Model file for the job. Use its own axes, mm. Face numbers are marked on the shaded views. A direction names the side the tool comes from. Coordinates: 2 decimals unless noted, no trailing zeros. Write each loop counter-clockwise with the first axis right and the second up, starting at its lowest first coordinate (ties: lowest second). Pieces come first, ordered by that corner, then holes.
Q1. Pull direction X, two halves, no side cores. Call the marked faces 5, 6 and 7: released by +X, released by -X, zero draft, split by the parting line, or undercut.
Q2. Band-saw the part on D-D, the plane y = -19.5. Write the cut outline in (x, z).
Q3. Band-saw the part on C-C, the plane x = -13.5. Write the cut outline in (y, z), plus the area to 3 significant figures.
Q4. Band-saw the part on B-B, the plane z = 7.5. Write the cut outline in (x, y).
Q5. Pin check, flat tips, straight feed: P1, Ø14.5, axis at x = -13, y = 9.5, coming from the +Z side; P2, Ø1.5, axis at y = -7, z = 7.5, coming from the +X side; P3, Ø1, axis at x = -4.5, z = 3, coming from the +Y side. Stop position of each tip, or through.
Q6. Band-saw the part on A-A, the plane y = -2.5. Write the cut outline in (x, z), plus the area to 3 significant figures.
Q7. Which spindle directions (+Z, -Z, +X, -X, +Y, -Y) get a long thin tool onto all of the face, cutting with end or side? Do the marked faces 1, 2, 3 and 4. Say none if no direction does.
Q8. Drill centre lines: probe 1 along X at (y, z) = (-3, 1.75); probe 2 along X at (y, z) = (-23, 4.5); probe 3 along Y at (x, z) = (-29.5, 8.5). Where is each one in solid material? Low to high.
from build123d import *

# Parameters (mm, degrees)
F0_W      = 90
F0_H      = 59.1
F0_R      = 1.55
F1_DEPTH  = 1.65
F2_W      = 63
F2_H      = 12
F3_DEPTH  = 3.2
F4_W      = 5
F4_H      = 5.5
F5_DEPTH  = 2.2
F6_W      = 2.23
F6_H      = 58.8
F6_W_2    = 3.77
F7_DEPTH  = 4.75
F8_W      = 15
F8_H      = 21
F9_DEPTH  = 1.3
F10_W     = 11.3
F10_H     = 4.5
F11_DEPTH = 3.85
F12_W     = 11
F12_H     = 7
F13_DEPTH = 7.5
F14_W     = 25
F14_H     = 25
F15_DEPTH = 10
F16_W     = 6
F16_H     = 10
F16_W_2   = 10
F16_H_2   = 1.2
F17_DEPTH = 4.75


with BuildPart() as f1:
    # F0 (on Top) → F1 (new body)
    with BuildSketch(Plane.XY):
        with Locations((-0.775745, -0.230454)):
            Rectangle(F0_W, F0_H)
        with Locations((-43.275745, -24.680454)):
            Circle(F0_R, mode=Mode.SUBTRACT)
        with Locations((36.224255, -25.980454)):
            Circle(F0_R, mode=Mode.SUBTRACT)
        with Locations((-42.525745, 26.569546)):
            Circle(F0_R, mode=Mode.SUBTRACT)
        with Locations((36.224255, 26.069546)):
            Circle(F0_R, mode=Mode.SUBTRACT)
    extrude(amount=F1_DEPTH)

    # F2 (on Top) → F3 (join)
    with BuildSketch(Plane.XY):
        Polygon((20.924255, -22.280454), (33.424255, -22.280454), (33.424255, 26.319546), (20.924255, 26.319546), (20.924255, 22.819546), (20.924255, 10.819546), align=None)
        with Locations((-10.575745, 16.819546)):
            Rectangle(F2_W, F2_H)
    extrude(amount=F3_DEPTH)

    # F4 (on face) → F5 (join)
    with BuildSketch(Plane.XY.offset(1.65)):
        with Locations((-33.275745, 25.569546)):
            Rectangle(F4_W, F4_H)
    extrude(amount=F5_DEPTH)

    # F6 (on face) → F7 (join)
    with BuildSketch(Plane.XY.offset(1.65)):
        with Locations((45.339255, -0.080454)):
            Rectangle(F6_W, F6_H)
        with Locations((42.339255, -0.080454)):
            Rectangle(F6_W_2, F6_H)
    extrude(amount=F7_DEPTH)

    # F8 (on face) → F9 (join)
    with BuildSketch(Plane.XY.offset(1.65)):
        with Locations((12.224255, -0.180454)):
            Rectangle(F8_W, F8_H)
    extrude(amount=F9_DEPTH)

    # F10 (on face) → F11 (join)
    with BuildSketch(Plane.XY.offset(1.65)):
        with Locations((25.574255, -25.530454)):
            Rectangle(F10_W, F10_H)
    extrude(amount=F11_DEPTH)

    # F12 (on face) → F13 (join)
    with BuildSketch(Plane.XY.offset(1.65)):
        with Locations((-34.275745, 5.836562)):
            Rectangle(F12_W, F12_H)
    extrude(amount=F13_DEPTH)

    # F14 (on face) → F15 (join)
    with BuildSketch(Plane.XY.offset(1.65)):
        with Locations((-18.275745, -16.780454)):
            Rectangle(F14_W, F14_H)
    extrude(amount=F15_DEPTH)

    # F16 (on face) → F17 (join)
    with BuildSketch(Plane.XY.offset(1.65)):
        with Locations((-42.775745, -3.480454)):
            Rectangle(F16_W, F16_H)
        Polygon((-40.775745, -24.980454), (-40.775745, -29.780454), (-30.775745, -29.780454), (-30.775745, -29.280454), (-30.775745, -24.980454), align=None)
        with Locations((-35.775745, -30.380454)):
            Rectangle(F16_W_2, F16_H_2)
    extrude(amount=F17_DEPTH)


solid = f1.part
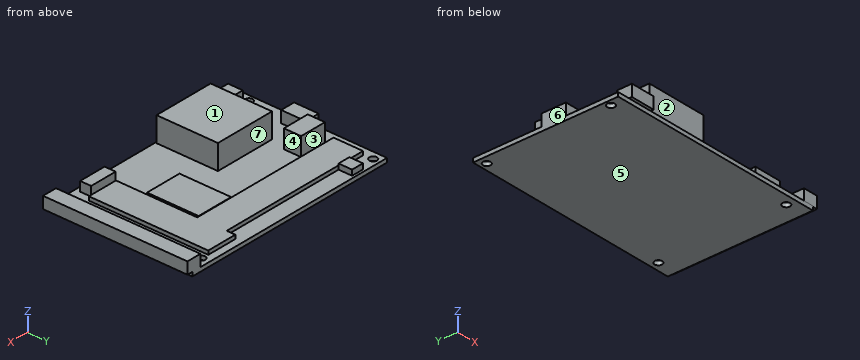
Answer sheet:
1. face 5: zero draft
1. face 6: released by -X
1. face 7: undercut
2. outline: (-45.78, 0) - (44.22, 0) - (44.22, 1.65) - (46.45, 1.65) - (46.45, 6.4) - (40.45, 6.4) - (40.45, 1.65) - (33.42, 1.65) - (33.42, 3.2) - (20.92, 3.2) - (20.92, 1.65) - (-5.78, 1.65) - (-5.78, 11.65) - (-30.78, 11.65) - (-30.78, 1.65) - (-45.78, 1.65) - close
3. outline: (-29.78, 0) - (29.32, 0) - (29.32, 1.65) - (22.82, 1.65) - (22.82, 3.2) - (10.82, 3.2) - (10.82, 1.65) - (-4.28, 1.65) - (-4.28, 11.65) - (-29.28, 11.65) - (-29.28, 1.65) - (-29.78, 1.65) - close
3. area: 366 mm2
4. outline: (-39.78, 2.34) - (-28.78, 2.34) - (-28.78, 9.34) - (-39.78, 9.34) - close; (-30.78, -29.28) - (-5.78, -29.28) - (-5.78, -4.28) - (-30.78, -4.28) - close
5. P1: stops at z = 3.2
5. P2: stops at x = -5.78
5. P3: stops at y = 22.82
6. outline: (-45.78, 0) - (44.22, 0) - (44.22, 1.65) - (46.45, 1.65) - (46.45, 6.4) - (40.45, 6.4) - (40.45, 1.65) - (33.42, 1.65) - (33.42, 3.2) - (20.92, 3.2) - (20.92, 1.65) - (19.72, 1.65) - (19.72, 2.95) - (4.72, 2.95) - (4.72, 1.65) - (-39.78, 1.65) - (-39.78, 6.4) - (-45.78, 6.4) - close
6. area: 244 mm2
7. face 1: +Z, +X, -X, +Y, -Y
7. face 2: +Z, -Y
7. face 3: +Z, -X
7. face 4: +Z
8. probe 1: x = -45.78 to -39.78, 4.72 to 19.72, 20.92 to 33.42, 40.45 to 46.45
8. probe 2: x = -30.78 to -5.78, 40.45 to 46.45
8. probe 3: y = -29.28 to -4.28, 2.34 to 9.34
